Here's how the part is built. I have some questions about the finished solid (model axes, mm). Face numbers are marked on the shaded views. Round coordinates to 2 decimals unless told otherwise and drop trailing zeros. Loops run counter-clockwise (first coordinate to the right, second up) from the corner with the lowest first, then second, coordinate; pieces in that order, holes last. Notation, with made-up numbers: M -6.75,64.25 L 4.25,64.25 A32 cw 4.25,100.25 Z; hole C 71.25,79 d7. An arc over 180 degrees is marked long. Answer as a JSON object with one key per item and string values.
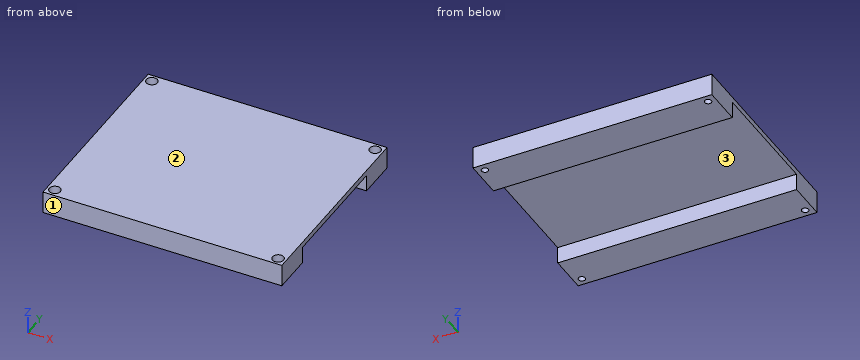
from build123d import *

# Parameters (mm, degrees)
SKETCH005_W                        = 107
SKETCH005_H                        = 90
PAD003_DEPTH                       = 10
SKETCH008_R                        = 2.5
POCKET004_DEPTH                    = 5
SKETCH009_R                        = 1.5
POCKET005_DEPTH                    = 285.350782
SKETCH008_LINEARPATTERN_2_R        = 2.5
POCKET004_LINEARPATTERN_2_DEPTH    = 5
LINEARPATTERN001_COUNT             = 2
LINEARPATTERN001_PITCH             = 83
SKETCH009_LINEARPATTERN002_2_R     = 1.5
POCKET005_LINEARPATTERN002_2_DEPTH = 285.350782
LINEARPATTERN003_COUNT             = 2
LINEARPATTERN003_PITCH             = 83
SKETCH012_W                        = 110
SKETCH012_H                        = 55
POCKET008_DEPTH                    = 7.5


with BuildPart() as part:
    # Sketch005 → Pad003 (new body)
    with BuildSketch(Plane.XY):
        with Locations((53.5, 45)):
            Rectangle(SKETCH005_W, SKETCH005_H)
    extrude(amount=PAD003_DEPTH)

    # Sketch008 (on Face6 of Pad003) → Pocket004 (cut)
    with BuildSketch(Plane.XY.offset(10)):
        with Locations((3.5, 86.5)):
            Circle(SKETCH008_R)
    pocket004 = extrude(amount=-POCKET004_DEPTH, mode=Mode.SUBTRACT)

    # Sketch009 (on Face8 of Pocket004) → Pocket005 (cut, through all)
    with BuildSketch(Plane.XY.offset(5)):
        with Locations((3.5, 86.5)):
            Circle(SKETCH009_R)
    pocket005 = extrude(amount=-POCKET005_DEPTH, mode=Mode.SUBTRACT)

    # Sketch008 LinearPattern 2 → Pocket004 LinearPattern 2 (cut)
    with BuildSketch(Plane(origin=(100, 0, 10), x_dir=(1, 0, 0), z_dir=(0, 0, 1))):
        with Locations((3.5, 86.5)):
            Circle(SKETCH008_LINEARPATTERN_2_R)
    pocket004_linearpattern_2 = extrude(amount=-POCKET004_LINEARPATTERN_2_DEPTH, mode=Mode.SUBTRACT)

    # LinearPattern001: Pocket004, Pocket004 LinearPattern 2 ×2
    with Locations(*[(0, -i * LINEARPATTERN001_PITCH, 0) for i in range(1, LINEARPATTERN001_COUNT)]):
        add(pocket004, mode=Mode.SUBTRACT)
        add(pocket004_linearpattern_2, mode=Mode.SUBTRACT)

    # Sketch009 LinearPattern002 2 → Pocket005 LinearPattern002 2 (cut, through all)
    with BuildSketch(Plane(origin=(100, 0, 5), x_dir=(1, 0, 0), z_dir=(0, 0, 1))):
        with Locations((3.5, 86.5)):
            Circle(SKETCH009_LINEARPATTERN002_2_R)
    pocket005_linearpattern002_2 = extrude(amount=-POCKET005_LINEARPATTERN002_2_DEPTH, mode=Mode.SUBTRACT)

    # LinearPattern003: Pocket005, Pocket005 LinearPattern002 2 ×2
    with Locations(*[(0, -i * LINEARPATTERN003_PITCH, 0) for i in range(1, LINEARPATTERN003_COUNT)]):
        add(pocket005, mode=Mode.SUBTRACT)
        add(pocket005_linearpattern002_2, mode=Mode.SUBTRACT)

    # Sketch012 (on Face4 of MultiTransform001) → Pocket008 (cut)
    with BuildSketch(Plane(origin=(0, 0, 0), x_dir=(1, 0, 0), z_dir=(0, 0, -1))):
        with Locations((53.5, -45)):
            Rectangle(SKETCH012_W, SKETCH012_H)
    extrude(amount=-POCKET008_DEPTH, mode=Mode.SUBTRACT)


with BuildPart() as part_1:
    # Body001 placement: moved
    add(part.part.moved(Location((0, 0, 30))))


solid = part_1.part
Item 1: I want a section at B-B, the plane x = 103.5. Please give me the cut outline in (y, z), then the cut area to 4 significant figures.
Resolved:
{"outline": "M 0,30 L 2,30 L 2,35 L 1,35 L 1,40 L 0,40 Z; M 5,30 L 17.5,30 L 17.5,37.5 L 72.5,37.5 L 72.5,30 L 85,30 L 85,35 L 84,35 L 84,40 L 6,40 L 6,35 L 5,35 Z; M 88,30 L 90,30 L 90,40 L 89,40 L 89,35 L 88,35 Z", "area": "407.5 mm²"}
Item 2: I want a section at A-A, the plane y = 3.5. Please give me the cut outline in (x, z).
Resolved:
{"outline": "M 0,30 L 2,30 L 2,35 L 1,35 L 1,40 L 0,40 Z; M 5,30 L 102,30 L 102,35 L 101,35 L 101,40 L 6,40 L 6,35 L 5,35 Z; M 105,30 L 107,30 L 107,40 L 106,40 L 106,35 L 105,35 Z"}
Item 3: Please list where these lines run through material, in increasing order: probe 1 along X at (y, z) = (86.5, 32.3); probe 2 along Y at (x, z) = (3.5, 37.45); probe 3 along Y at (x, z) = (56, 32.75). Write a range as from..to.
Resolved:
{"probe 1": "0..2, 5..102, 105..107", "probe 2": "0..1, 6..17.5, 72.5..84, 89..90", "probe 3": "0..17.5, 72.5..90"}
Item 4: I want a section at C-C, the plane x = 34.5. Please give me the cut outline in (y, z), then the cut area to 4 significant figures.
Resolved:
{"outline": "M 0,30 L 17.5,30 L 17.5,37.5 L 72.5,37.5 L 72.5,30 L 90,30 L 90,40 L 0,40 Z", "area": "487.5 mm²"}
Item 5: If we mould it in two halves opening along Y, with no side actions, what happens to the marked faces 1, 2 and 3? For each: pulls with the +Y half, pulls with the -Y half, needs draft (parallel to the pull), parting line crosses it, or undercut.
Resolved:
{"face 1": "pulls with the -Y half", "face 2": "needs draft", "face 3": "undercut"}
Item 6: I want a section at D-D, the plane y = 56. Please give me the cut outline in (x, z).
Resolved:
{"outline": "M 0,37.5 L 107,37.5 L 107,40 L 0,40 Z"}
Item 7: I'm going to push flat-ended pins straight in: pin 1 Ø2.5 at (x, y) = (3.5, 87) entering from +Z; pin 2 Ø1 at (x, y) = (77.5, 58) entering from -Z. Where does each tip first touch, or does it pass through?
Resolved:
{"pin 1": "z = 35", "pin 2": "z = 37.5"}
